```python
from build123d import *

# Parameters (mm, degrees)
F0_W     = 2.00000108
F0_H     = 20.0000108
F2_R     = 18.19299892
F3_DEPTH = 2.00000108
F4_R     = 1.5875


# Not quite as in the source:
# - a fillet or chamfer that OpenCascade refuses, or shapes differently, is made with other operations: its cross-section is extruded or revolved along the edge and cut away or added


with BuildPart() as f1:
    # F0 (on Front) → F1 (revolve)
    with BuildSketch(Plane.XZ):
        with Locations((19.19299946, 10.0000054)):
            Rectangle(F0_W, F0_H)
        Polygon((30.48659892, 69.9999108), (18.19299892, 20.0000108), (20.193, 20.0000108), (21.19299292, 20.0000108), (33.48659292, 69.9999108), (32.4866, 69.9999108), align=None)
        with Locations((31.48659946, 79.9999162)):
            Rectangle(F0_W, F0_H)
    revolve(axis=Axis((0, 0, 12.2811223036), (0, 0, 1)))

    # F2 (on Top) → F3 (join)
    with BuildSketch(Plane.XY):
        Circle(F2_R)
    extrude(amount=F3_DEPTH)

    # F4
    f4_edges = [f1.edges().sort_by_distance(p)[0] for p in [
        (-20.193, 0, 0),
    ]]
    fillet(f4_edges, radius=F4_R)

    # F5: fillet of radius 3.175 on 1 edges, made by hand

    # F5_s1 → F5_t2 (revolve, cut)
    with BuildSketch(Plane.XZ):
        with BuildLine():
            ThreePointArc((32.4866, 87.050344929), (31.9394552634, 88.8321983782), (30.48659892, 89.9999216))
            Line((30.48659892, 89.9999216), (32.4866, 89.9999216))
            Line((32.4866, 89.9999216), (32.4866, 87.050344929))
        make_face()
    revolve(axis=Axis((0, 0, 89.9999216), (0, 0, 1)), mode=Mode.SUBTRACT)


solid = f1.part
```
Input: part model. Units: mm. Frame: model coordinates. A direction names the side the tool comes from. Round coordinates to 2 decimals unless told otherwise and drop trailing zeros. Loops run counter-clockwise (first coordinate to the right, second up) from the corner with the lowest first, then second, coordinate; pieces in that order, holes last. Notation, with made-up numbers: (-27.75, -17.5) -> (27.25, -17.5) arc R13 cw to (27.25, -11.5) -> close; hole circle Ø11 at (-29.5, 30.25). An arc over 180 degrees is marked (long way). Use one line per item in the form item = value. Start each with the question number.
Item 1: Section query C-C on z = 10.5. Return the cut outline in (x, y), then the cut area to 3 significant figures.
Item 2: Set-up query: faces 4 (the face through (0, 0, 0)), 5 (the face through (-2.63, 20.02, 10.92)), 6 (the face through (29.08, 9.16, 80.14)). Return all of +Z, -Z, +X, -X, +Y, -Y with unobstructed straight access to the full face (end or side cutting, diameter ignored); none if empty.
Item 3: Mould query, pull axis Y, two halves, no side actions, for faces 1 (the face through (-2.98, 22.69, 39.09)), 2 (the face through (-5.1, 32.4, 70)), 3 (the face through (-5.65, -25.44, 39.79)). Classes: pulls with the +Y half, pulls with the -Y half, needs draft (parallel to the pull), parting line crosses it, or undercut.
Item 4: Section query D-D on z = 65. Return the cut outline in (x, y).
Item 5: Material intervals for L1, parallel to Y at x = 0, z = 6.5; L2, parallel to Y at x = 0, z = 82; L3, parallel to Z at x = 1, y = -12, sorted ascending. Write a range as from..to.
Item 6: Contact query for flat-ended pins moving along their axis: pin 1 Ø1 at (y, z) = (-2.5, 26) entering from -X; pin 2 Ø10 at (y, z) = (-26, 46) entering from +X; pin 3 Ø4 at (y, z) = (-8, 33) entering from +X; pin 4 Ø8 at (x, y) = (21.5, -23.5) entering from +Z. Output: stop coordinate, or through.
Ans:
q1.outline = circle Ø40.39 at (0, 0); hole circle Ø36.39 at (0, 0)
q1.area = 241 mm^2
q2.face_4 = -Z, +X, -X, +Y, -Y
q2.face_5 = -Z
q2.face_6 = +Z
q3.face_1 = undercut
q3.face_2 = needs draft
q3.face_3 = parting line crosses it
q4.outline = circle Ø64.51 at (0, 0); hole circle Ø58.51 at (0, 0)
q5.L1 = -20.19..-18.19, 18.19..20.19
q5.L2 = -32.49..-30.49, 30.49..32.49
q5.L3 = 0..2
q6.pin_1 = -22.66
q6.pin_2 = 18.19
q6.pin_3 = 23.84
q6.pin_4 = 90
